```python
from build123d import *

# Parameters (mm, degrees)
CHAMFER1_SIZE = 0.5


with BuildPart() as part:
    # Sketch1 → Revolve1 (revolve)
    with BuildSketch(Plane.XY):
        Polygon((15, 0), (16.512706206, 0), (16.512706206, 0.048438063), (25.873387513, 0.048438063), (25.873387513, 0), (29.125, 0), (29.125, 3.25), (27.5, 3.25), (27.5, 13), (25.873387513, 13), (25.873387513, 12.951561937), (16.512706206, 12.951561937), (16.512706206, 13), (15, 13), align=None)
    revolve(axis=Axis((0, 0, 0), (0, 1, 0)))

    # Chamfer1
    chamfer1_edges = [part.edges().sort_by_distance(p)[0] for p in [
        (-29.125, 0, 0),
    ]]
    chamfer(chamfer1_edges, length=CHAMFER1_SIZE)


solid = part.part
```
The listing builds one solid part. Answer for the finished solid, in the listing's coordinates (mm). A direction names the side the tool comes from. Round coordinates to 2 decimals unless told otherwise and drop trailing zeros. Loops run counter-clockwise (first coordinate to the right, second up) from the corner with the lowest first, then second, coordinate; pieces in that order, holes last.
1) Consider line 1 (Z direction, x = 0, y = 10.25); line 2 (Y direction, x = -22.5, z = 7); line 3 (X direction, y = 2, z = 10.5). Determine where each line is inside the solid, lowest interval first.
Outcome:
line 1: z = -27.5 to -15, 15 to 27.5
line 2: y = 0.05 to 12.95
line 3: x = -27.17 to -10.71, 10.71 to 27.17
2) A cutting plane is placed at C-C on y = 7. Determine the outline of the cut face in (x, z).
Outcome:
outline: circle Ø55 at (0, 0); hole circle Ø30 at (0, 0)
3) For faces 4 (the face through (6.5, 0, 25.3)), 5 (the face through (11, 3.25, 26)), determine the directions among +Z, -Z, +X, -X, +Y, -Y from which every point of the face is accessible in a straight line to the end or side of a thin tool.
Outcome:
face 4: +Z, -Z, +X, -X, -Y
face 5: +Y
4) Given P1, Ø1.5, axis at y = 3.5, z = 21, coming from the +X side; P2, Ø4, axis at x = 19, z = -0.5, coming from the -Y side; P3, Ø3, axis at x = -16.5, y = 7.5, coming from the -Z side; P4, Ø2, axis at x = 10.5, z = 9, coming from the -Y side, each flat-ended and moving along its own axis, determine where each tip first touches the part or whether it passes through.
Outcome:
P1: stops at x = 20.89
P2: stops at y = 0.05
P3: stops at z = -23.05
P4: passes through
5) For a pull along Z with two mould halves and no side action, classify faces 1 (the face through (-14.985, 6.409, -0.66)), 2 (the face through (4, 13, 15)), 3 (the face through (-5.961, 8.193, 26.846)) as released by +Z, released by -Z, zero draft, split by the parting line, or undercut.
Outcome:
face 1: undercut
face 2: zero draft
face 3: split by the parting line
